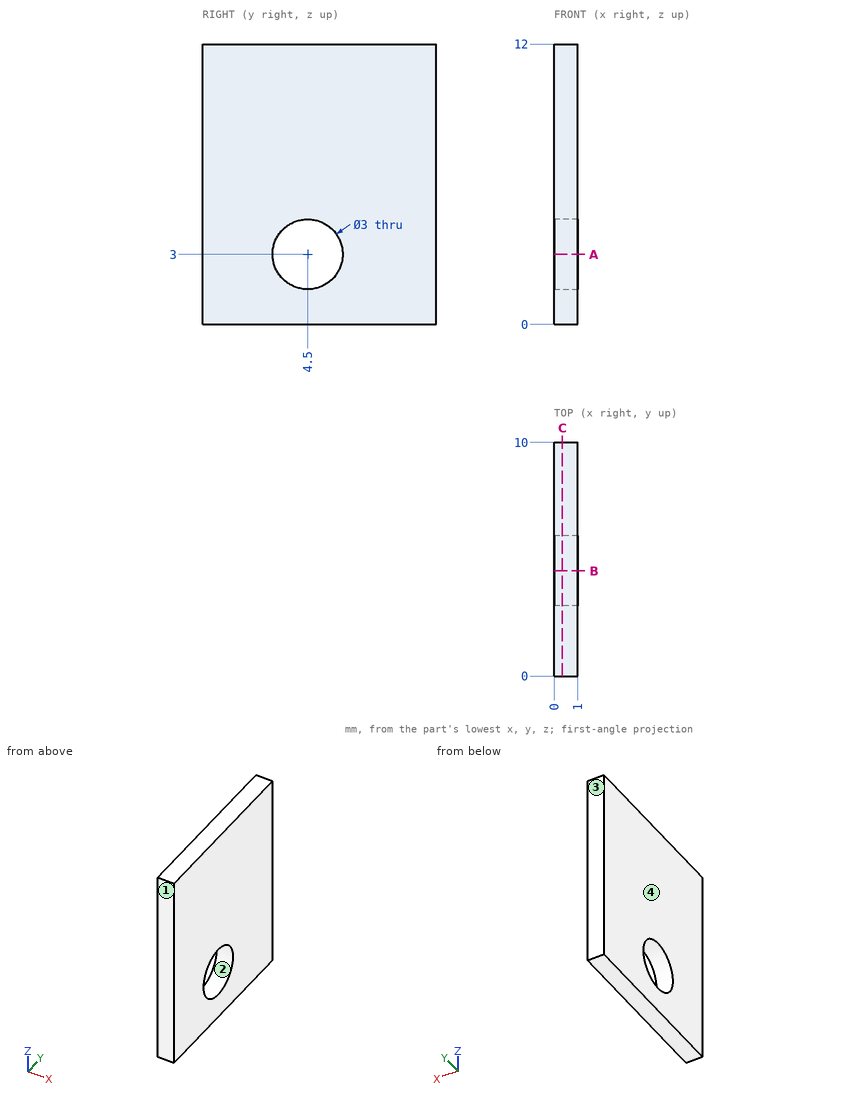
Design review of the part shown in the three views and the two pictorial views. Dimensions are in mm from the part's minimum x, y and z. Give positions to 0.01 mm unless a question says otherwise; leave off trailing zeros. Loops run counter-clockwise (first coordinate to the right, second up) from the corner with the lowest first, then second, coordinate; pieces in that order, holes last. Notation, with made-up numbers: (88, -35) -> (125, -35) arc R23 ccw to (125, -13) -> close; hole circle Ø3 at (29.5, 6). An arc over 180 degrees is marked (long way). Answer as a JSON object with one key per item and string values. Group by question number.
Q1. Take a section at C-C (x = 0.35). Write out the cut boundary in (y, z).
Q2. Take a section at B-B (y = 4.5). Write out the cut boundary in (x, z), plus the area to 3 significant figures.
Q3. Take a section at A-A (z = 3). Write out the cut boundary in (x, y), plus the area to 3 significant figures.
Q4. Draft analysis for pull direction Y (two halves, no side actions). For the marked faces 1, 2, 3 and 4, state which applies: pulls with the +Y half, pulls with the -Y half, needs draft (parallel to the pull), parting line crosses it, or undercut.
Q5. Wall thickness on line 1 along Y through (x, z) = (0.65, 3); line 2 along Z through (x, y) = (0.2, 4.5); line 3 along Z through (x, y) = (0.25, 5.75): over which ranges is each line inside the solid? List them lowest first.
Answer below:
{
 "1": {"outline": "(0, 0) -> (10, 0) -> (10, 12) -> (0, 12) -> close; hole circle Ø3 at (4.5, 3)"},
 "2": {"outline": "(0, 0) -> (1, 0) -> (1, 1.5) -> (0, 1.5) -> close; (0, 4.5) -> (1, 4.5) -> (1, 12) -> (0, 12) -> close", "area": "9.00 mm2"},
 "3": {"outline": "(0, 0) -> (1, 0) -> (1, 3) -> (0, 3) -> close; (0, 6) -> (1, 6) -> (1, 10) -> (0, 10) -> close", "area": "7.00 mm2"},
 "4": {"face 1": "pulls with the -Y half", "face 2": "undercut", "face 3": "pulls with the +Y half", "face 4": "needs draft"},
 "5": {"line 1": "y = 0 to 3, 6 to 10", "line 2": "z = 0 to 1.5, 4.5 to 12", "line 3": "z = 0 to 2.17, 3.83 to 12"}
}
